The listing builds one solid part. Answer for the finished solid, in the listing's coordinates (mm). A direction names the side the tool comes from. Round coordinates to 2 decimals unless told otherwise and drop trailing zeros. Loops run counter-clockwise (first coordinate to the right, second up) from the corner with the lowest first, then second, coordinate; pieces in that order, holes last. Notation, with made-up numbers: M 37.5,29 L 83.5,29 A10 ccw 83.5,38 Z; hole C 62,-31 d5. An arc over 180 degrees is marked long. Put each result on its own line as item: value. Start each with the question number.
(1) Section C-C, the plane y = 0.65 is taken. Determine the outline of the cut face in (x, z) (3 decimals).
(2) Section B-B, the plane x = -7 is taken. Determine the outline of the cut face in (y, z) (3 decimals).
(3) Determine the mould class of faces 3 (the face through (-20, 1, 0)), 4 (the face through (9, 1, -6.012)), 5 (the face through (0, 1, -20)) for opening direction X: released by +X, released by -X, zero draft, split by the parting line, or undercut.
(4) Which of the six approach directions +Z, -Z, +X, -X, +Y, -Y give full straight-line access (tool end or side, diameter ignored) to faces 1 (the face through (0, 0, 0)), 2 (the face through (9, 1, 5.988))?
(5) Section A-A, the plane z = 0 is taken. Determine the outline of the cut face in (x, y) (3 decimals).
(6) Section D-D, the plane x = 16.5 is taken. Determine the outline of the cut face in (y, z), then the cut area to 3 significant figures.
(7) A flat-ended cylindrical pin translates along its axis: P1, Ø2.5, axis at x = -15.22, z = -15.22, coming from the -Y side. Find the tip coordinate at first contact, or state that the pin passes through.
(8) Straight lines are drawn through the part: line 1 (X direction, y = 2.85, z = -13.5); line 2 (Z direction, x = -16, y = 0.75). For each, find the intervals that lie inside material, in ascending order.
```python
from build123d import *

# Parameters (mm, degrees)
SKETCH_2_W          = 40
SKETCH_2_H          = 40
EXTRUDE_2_DEPTH     = 3
SKETCH_3_R          = 2
SKETCH_3_R_2        = 5.125
SKETCH_3_W          = 3
SKETCH_3_H          = 12
CUT_EXTRUDE_1_DEPTH = 3


with BuildPart() as part:
    # 草图2 → 凸台-拉伸2 (new body)
    with BuildSketch(Plane(origin=(0, 0, 0), x_dir=(1, 0, 0), z_dir=(0, 1, 0))):
        Rectangle(SKETCH_2_W, SKETCH_2_H)
    extrude(amount=EXTRUDE_2_DEPTH)

    # 草图3 → 切除-拉伸1 (cut)
    with BuildSketch(Plane(origin=(0, 0, 0), x_dir=(1, 0, 0), z_dir=(0, 1, 0))):
        with Locations(Location((-15.224798987, -15.224798987, 0), (0, 0, 270))):
            Circle(SKETCH_3_R)
        with Locations(Location((15.224798987, -15.224798987, 0), (0, 0, 270))):
            Circle(SKETCH_3_R)
        with Locations(Location((15.224798987, 15.224798987, 0), (0, 0, 270))):
            Circle(SKETCH_3_R)
        with Locations(Location((-15.224798987, 15.224798987, 0), (0, 0, 270))):
            Circle(SKETCH_3_R)
        with Locations(Location((-7, 0, 0), (0, 0, 270))):
            Circle(SKETCH_3_R_2)
        with Locations((9.5, 0.011605537)):
            Rectangle(SKETCH_3_W, SKETCH_3_H)
    extrude(amount=CUT_EXTRUDE_1_DEPTH, mode=Mode.SUBTRACT)


solid = part.part
```
Recorded:
1. outline: M -20,-20 L 20,-20 L 20,20 L -20,20 Z; hole C -15.225,-15.225 d4; hole C -15.225,15.225 d4; hole C -7,0 d10.25; hole M 8,-6.012 L 11,-6.012 L 11,5.988 L 8,5.988 Z; hole C 15.225,-15.225 d4; hole C 15.225,15.225 d4
2. outline: M 0,-20 L 3,-20 L 3,-5.125 L 0,-5.125 Z; M 0,5.125 L 3,5.125 L 3,20 L 0,20 Z
3. face 3: released by -X
3. face 4: undercut
3. face 5: zero draft
4. face 1: +Z, -Z, +X, -X, -Y
4. face 2: +Y, -Y
5. outline: M -20,0 L -12.125,0 L -12.125,3 L -20,3 Z; M -1.875,0 L 8,0 L 8,3 L -1.875,3 Z; M 11,0 L 20,0 L 20,3 L 11,3 Z
6. outline: M 0,-20 L 3,-20 L 3,-16.77 L 0,-16.77 Z; M 0,-13.68 L 3,-13.68 L 3,13.68 L 0,13.68 Z; M 0,16.77 L 3,16.77 L 3,20 L 0,20 Z
6. area: 102 mm²
7. P1: passes through
8. line 1: x = -20 to -16.24, -14.21 to 14.21, 16.24 to 20
8. line 2: z = -20 to -17.07, -13.38 to 13.38, 17.07 to 20
